from build123d import *

# Parameters (mm, degrees)
F0_R     = 8.5
F1_DEPTH = 4
F2_R     = 5
F3_DEPTH = 100
F6_R     = 1.5
F7_DEPTH = 133.7


with BuildPart() as f1:
    # F0 (on Top) → F1 (new body)
    with BuildSketch(Plane.XY):
        Circle(F0_R)
    extrude(amount=F1_DEPTH)

    # F2 (on Top) → F3 (join)
    with BuildSketch(Plane.XY):
        Circle(F2_R)
    extrude(amount=F3_DEPTH)

    # F4 (on Right) → F5 (revolve)
    with BuildSketch(Plane.YZ):
        with BuildLine():
            Line((0, 100), (5, 100))
            ThreePointArc((5, 100), (3.535534, 103.535534), (0, 105))
            Line((0, 105), (0, 100))
        make_face()
    revolve(axis=Axis((0, 0, 102.5), (0, 0, -1)))

    # F6 (on face) → F7 (cut)
    with BuildSketch(Plane(origin=(0, 0, 0), x_dir=(1, 0, 0), z_dir=(0, 0, -1))):
        Circle(F6_R)
    extrude(amount=-F7_DEPTH, mode=Mode.SUBTRACT)


solid = f1.part
Work out the finished part from the listing and answer in its coordinate system (mm). Coordinates: 2 decimals unless noted, no trailing zeros. Loops run counter-clockwise (first coordinate to the right, second up) from the corner with the lowest first, then second, coordinate; pieces in that order, holes last. Notation, with made-up numbers: M -11,39.5 L 15,39.5 A26 cw 15,74.5 Z; hole C 64.25,84.25 d1. An arc over 180 degrees is marked long. Answer in a Markdown table with one row per item. Add a question column.
1. Find section B-B, the plane x = -6.5. Write down the section's boundary in (y, z).
2. Find section C-C, the plane y = -7. Write down the section's boundary in (x, z).
3. The mould has two halves that part along Y. Classify faces 1 (the cylindrical face through (-1.08, -4.88, 51.33)), 2 (the cylindrical face through (-1.5, -0.07, 51.65)), 3 (the flat face through (4, -4, 4)): pulls with the +Y half, pulls with the -Y half, needs draft (parallel to the pull), parting line crosses it, or undercut.
4. Consider L1, parallel to X at y = 0, z = 83; L2, parallel to Z at x = -3, y = 5.5. Determine where each line is inside the solid, lowest interval first.
5. Find section A-A, the plane z = 11. Write down the section's boundary in (x, y), then the cut area to 3 significant figures.
6. Flat-ended cylindrical pins translate along their axes: P1, Ø6, axis at x = 2.5, y = 1, coming from the +Z side; P2, Ø3, axis at x = 1, z = 68.5, coming from the +Y side; P3, Ø4, axis at y = 4, z = 41.5, coming from the -X side; P4, Ø2, axis at x = -2.5, z = 23, coming from the +Y side. Find the tip coordinate at first contact, or state that the pin passes through.
Reported:
| question | item | result |
|---|---|---|
| 1 | outline | M -5.48,0 L 5.48,0 L 5.48,4 L -5.48,4 Z |
| 2 | outline | M -4.82,0 L 4.82,0 L 4.82,4 L -4.82,4 Z |
| 3 | face 1 | parting line crosses it |
| 3 | face 2 | undercut |
| 3 | face 3 | needs draft |
| 4 | L1 | x = -5 to -1.5, 1.5 to 5 |
| 4 | L2 | z = 0 to 4 |
| 5 | outline | C 0,0 d10; hole C 0,0 d3 |
| 5 | area | 71.5 mm^2 |
| 6 | P1 | stops at z = 104.77 |
| 6 | P2 | stops at y = 5 |
| 6 | P3 | stops at x = -4.58 |
| 6 | P4 | stops at y = 4.77 |
